Can you work these out from the model? Positions are in its coordinate system, mm. Face numbers are marked on the shaded views. A direction names the side the tool comes from. Round coordinates to 2 decimals unless told otherwise and drop trailing zeros. Loops run counter-clockwise (first coordinate to the right, second up) from the corner with the lowest first, then second, coordinate; pieces in that order, holes last. Notation, with made-up numbers: M -22.75,-30.5 L 20.25,-30.5 A5 cw 20.25,-21.5 Z; hole C 72,75.25 d8. An arc over 180 degrees is marked long. Use a Markdown table: item, result. Add a question column.
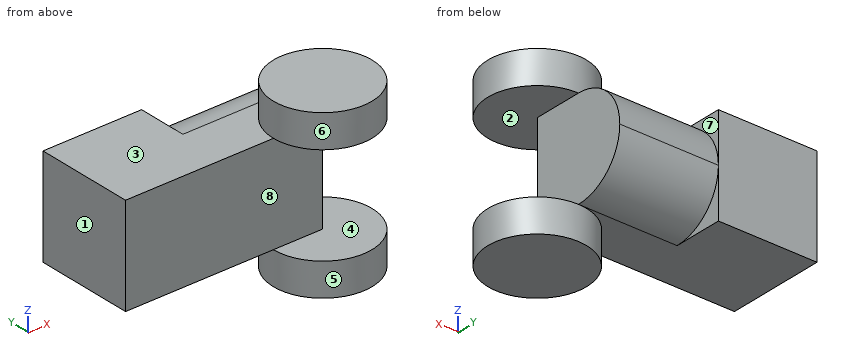
```python
from build123d import *

# Parameters (mm, degrees)
F0_W     = 38.1
F0_H     = 38.1
F1_DEPTH = 38.1
F3_DEPTH = 38.1
F4_DEPTH = 19.05
F7_DEPTH = 12.7
F8_DEPTH = 12.7


# Not quite as in the source:
# - a feature of the source that left no trace in its solid (it failed there, or was rolled back) is left out


with BuildPart() as f1:
    # F0 (on Front) → F1 (new body)
    with BuildSketch(Plane.XZ):
        with Locations((-45.594806087, -5.8171211302)):
            Rectangle(F0_W, F0_H)
    extrude(amount=F1_DEPTH)

    # F2 (on face) → F3 (join)
    with BuildSketch(Plane.YZ.offset(-26.544806087)):
        with BuildLine():
            Line((-19.05, 13.2328788698), (-19.05, -24.8671211302))
            ThreePointArc((-19.05, -24.8671211302), (-5.5796158184, -19.2875053118), (0, -5.8171211302))
            ThreePointArc((0, -5.8171211302), (-5.5796158184, 7.6532630514), (-19.05, 13.2328788698))
        make_face()
    extrude(amount=F3_DEPTH)

    # F4 (add): a face of the model
    f4_faces = [f1.faces().sort_by_distance(p)[0] for p in [
        (-7.494806087, -19.05, -5.8171211302),
    ]]
    extrude(f4_faces, amount=F4_DEPTH)

    # F6 (on face) → F7 (join)
    with BuildSketch(Plane.XY.offset(13.2328788698)):
        with BuildLine():
            ThreePointArc((-7.494806087, -38.1), (11.555193913, -57.15), (30.605193913, -38.1))
            ThreePointArc((30.605193913, -38.1), (25.0255780946, -24.6296158184), (11.555193913, -19.05))
            Line((11.555193913, -19.05), (11.555193913, -38.1))
            Line((11.555193913, -38.1), (-7.494806087, -38.1))
        make_face()
        with BuildLine():
            Line((11.555193913, -38.1), (11.555193913, -19.05))
            ThreePointArc((11.555193913, -19.05), (-1.9151902686, -24.6296158184), (-7.494806087, -38.1))
            Line((-7.494806087, -38.1), (11.555193913, -38.1))
        make_face()
    extrude(amount=F7_DEPTH)

    # F5 (on face) → F8 (join)
    with BuildSketch(Plane(origin=(0, 0, -24.8671211302), x_dir=(1, 0, 0), z_dir=(0, 0, -1))):
        with BuildLine():
            Line((11.555193913, 38.1), (11.555193913, 19.05))
            ThreePointArc((11.555193913, 19.05), (25.0255780946, 24.6296158184), (30.605193913, 38.1))
            ThreePointArc((30.605193913, 38.1), (11.555193913, 57.15), (-7.494806087, 38.1))
            Line((-7.494806087, 38.1), (11.555193913, 38.1))
        make_face()
        with BuildLine():
            ThreePointArc((-7.494806087, 38.1), (-1.9151902686, 24.6296158184), (11.555193913, 19.05))
            Line((11.555193913, 19.05), (11.555193913, 38.1))
            Line((11.555193913, 38.1), (-7.494806087, 38.1))
        make_face()
    extrude(amount=F8_DEPTH)


solid = f1.part
```
(1) If I drill on probe 1 along Z at (x, y) = (23, -24.5); probe 2 along X at (y, z) = (-28.5, 12.5); probe 3 along X at (y, z) = (-4, -19.5), over which ranges is the centre line in solid material (lowest first)? Write a range as [from, to].
(2) I'm going to push flat-ended pins straight in: pin 1 (12 mm diameter, centred on x = -10.5, z = -13.5, fed in from +Y); pin 2 (6 mm diameter, centred on y = -30.5, z = 6, fed in from +X); pin 3 (1 mm diameter, centred on x = -35.5, y = -16.5, fed in from -Z). Where does each tip first touch, or does it pass through?
(3) Thinking about a two-plate mould opening in Z: for the marked faces 1, 2 and 3, which applies, released by +Z, released by -Z, zero draft, split by the parting line, or undercut?
(4) Suppose I cut it at B-B on x = -18. List the corners of the cut face in (y, z) for me, and give its area (3 significant figures).
(5) Suppose I cut it at C-C on y = -25. List the corners of the cut face in (x, z) for me, and give its area (3 significant figures).
(6) On a 3-axis mill with a long thin cutter (end or side, diameter ignored), from which of +Z, -Z, +X, -X, +Y, -Y can I reach the whole of each face in a straight line? I mean the marked faces 4, 5, 6, 7 and 8. Say none if no direction works.
(7) Suppose I cut it at A-A on y = -50. List the corners of the cut face in (x, z) for me.
(8) Suppose I cut it at D-D on z = -33. List the corners of the cut face in (x, y) for me.
Results below:
| question | item | result |
|---|---|---|
| 1 | probe 1 | z = [-37.57, -24.87], [13.23, 25.93] |
| 1 | probe 2 | x = [-64.64, 11.56] |
| 1 | probe 3 | x = [-64.64, -26.54] |
| 2 | pin 1 | stops at y = -0.07 |
| 2 | pin 2 | stops at x = 11.56 |
| 2 | pin 3 | stops at z = -24.87 |
| 3 | face 1 | zero draft |
| 3 | face 2 | undercut |
| 3 | face 3 | released by +Z |
| 4 | outline | M -38.1,-24.87 L -19.05,-24.87 A19.05 ccw -19.05,13.23 L -38.1,13.23 Z |
| 4 | area | 1,300 mm² |
| 5 | outline | M -64.64,-24.87 L -2.28,-24.87 L -2.28,-37.57 L 25.39,-37.57 L 25.39,-24.87 L 11.56,-24.87 L 11.56,13.23 L 25.39,13.23 L 25.39,25.93 L -2.28,25.93 L -2.28,13.23 L -64.64,13.23 Z |
| 5 | area | 3,610 mm² |
| 6 | face 4 | +X, -Y |
| 6 | face 5 | -Z |
| 6 | face 6 | +Z |
| 6 | face 7 | +Z, +X, +Y |
| 6 | face 8 | +X, -X, -Y |
| 7 | outline | M -3.32,-37.57 L 26.43,-37.57 L 26.43,-24.87 L -3.32,-24.87 Z; M -3.32,13.23 L 26.43,13.23 L 26.43,25.93 L -3.32,25.93 Z |
| 8 | outline | C 11.56,-38.1 d38.1 |
